Autodesk Inventor part; units mm, degrees
ref_plane "YZ Plane" through (0, 0, 0) normal (1, 0, 0) x (0, 1, 0)
ref_plane "XZ Plane" through (0, 0, 0) normal (0, 1, 0) x (-1, 0, 0)
ref_plane "XY Plane" through (0, 0, 0) normal (0, 0, 1) x (1, 0, 0)
sketch "Sketch1" plane through (0, 0, 0) normal (1, 0, 0) x (0, 1, 0)
  line L0 (0, 0) -> (76.2, 0)
  line L1 (76.2, 0) -> (76.2, -863.6)
  line L2 (76.2, -863.6) -> (0, -863.6)
  line L3 (0, -863.6) -> (0, 0)
  dimension "d0" = 76.2
  dimension "d1" = 863.6
extrude "Extrusion1" add sketch "Sketch1" along normal blind 3.175
sketch "Sketch2" plane through (3.175, 0, 0) normal (1, 0, 0) x (0, 0, -1)
  line L0 (0, 38.1) -> (0, 36.5125)
  line L1 (0, 36.5125) -> (0, 39.6875)
  circle A0 centre (306.07, 36.5125) radius 14.2875
  circle A1 centre (557.53, 36.5125) radius 14.2875
  circle A2 centre (105.4351, 39.6875) radius 14.2875
  circle A3 centre (758.1649, 39.6875) radius 14.2875
  line L2 (863.6, 0) -> (838.2, 0)
  line L3 (863.6, 0) -> (863.6, 38.1)
  line L4 (863.6, 38.1) -> (838.2, 0)
  circle A4 centre (12.7, 63.5) radius 3.175
  line L5 (863.6, 76.2) -> (0, 76.2)
  circle A5 centre (850.9, 63.5) radius 3.175
  circle A6 centre (825.5, 15.875) radius 3.175
  circle A7 centre (38.1, 15.875) radius 3.175
  circle A8 centre (190.5, 15.875) radius 3.175
  circle A9 centre (431.8, 15.875) radius 3.175
  circle A10 centre (431.8, 63.5) radius 3.175
  circle A11 centre (673.1, 63.5) radius 3.175
  circle A12 centre (673.1, 15.875) radius 3.175
  circle A13 centre (190.5, 63.5) radius 3.175
  line L6 (0, 0) -> (25.4, 0)
  line L7 (0, 0) -> (0, 38.1)
  line L8 (0, 38.1) -> (25.4, 0)
  line L9 (863.6, 0) -> (0, 0)
  dimension "d15" = 28.575
  dimension "d16" = 28.575
  dimension "d19" = 28.575
  dimension "d21" = 28.575
  dimension "d22" = 25.4
  dimension "d26" = 6.35
  dimension "d27" = 12.7
  dimension "d29" = 6.35
  dimension "d30" = 12.7
  dimension "d32" = 6.35
  dimension "d34" = 12.7
  dimension "d35" = 6.35
  dimension "d39" = 6.35
  dimension "d40" = 863.6
  dimension "d41" = 6.35
  dimension "d43" = 6.35
  dimension "d44" = 12.7
  dimension "d45" = 6.35
  dimension "d46" = 6.35
  dimension "d48" = 241.3
  dimension "d49" = 241.3
  dimension "d50" = 6.35
  dimension "d51" = 241.3
  dimension "d53" = 241.3
  dimension "d54" = 25.4
  dimension "d55" = 38.1
  dimension "d58" = 15.875
  dimension "d59" = 15.875
  dimension "d60" = 15.875
extrude "Extrusion3" cut sketch "Sketch2" against normal blind 25.4
properties part number "OutsidePlate"
Geometry check sheet. Reference: the model listing, model coordinates, mm. Round coordinates to 2 decimals unless told otherwise and drop trailing zeros. Order: outer loops, then holes, each group sorted by start corner. A loop starts at its lowest first (then second) coordinate and runs counter-clockwise, first axis right, second up. Notation, with made-up numbers: (-27.75, 33.5) -> (1.25, 33.5) arc R11 cw to (1.25, 42.5) -> close; hole circle Ø8 at (-11, 82.5). An arc over 180 degrees is marked (long way). Use one line per item in the form item = value.
1. Cross-section at A-A, the plane z = -306.07. Enter the section's corners in (x, y) (3 decimals), plus the area to 3 significant figures.
Working result:
outline = (0, 0) -> (3.175, 0) -> (3.175, 22.225) -> (0, 22.225) -> close; (0, 50.8) -> (3.175, 50.8) -> (3.175, 76.2) -> (0, 76.2) -> close
area = 151 mm^2
2. Mould release check, pull along Z, two halves, no side actions. Record for faces 1 (the face through (1.61, 37.141, -543.256)), 2 (the face through (0, 38, -426)), 3 (the face through (1.61, 19.32, -851.08)): pulls with the +Z half, pulls with the -Z half, needs draft (parallel to the pull), parting line crosses it, or undercut.
Working result:
face_1 = undercut
face_2 = needs draft
face_3 = pulls with the -Z half
3. Scan lines: line 1 along Y through (x, z) = (1, -190.5) (3 decimals); line 2 along Y through (x, z) = (1.35, -825.5); line 3 along Z through (x, y) = (0.1, 32). Record each from-to range of solid material in increasing order. Write a range as from..to.
Working result:
line_1 = 0..12.7, 19.05..60.325, 66.675..76.2
line_2 = 0..12.7, 19.05..76.2
line_3 = -859.53..-770.21, -746.12..-571.09, -543.97..-319.63, -292.51..-117.48, -93.39..-4.07
4. Cross-section at B-B, the plane x = 0.6. Count the separate pieces of the cut face and the enclosed holes in it, plus the area to 3 significant figures.
Working result:
separate_pieces = 1
enclosed_holes = 14
area = 62,000 mm^2
5. Go/stop test with flat-tipped pins: pin 1 (10 mm diameter, centred on y = 15.875, z = -825.5, fed in from -X); pin 2 (5.5 mm diameter, centred on y = 15.875, z = -431.8, fed in from +X). Record where each tip stops, or that it passes through.
Working result:
pin_1 = 0
pin_2 = through
